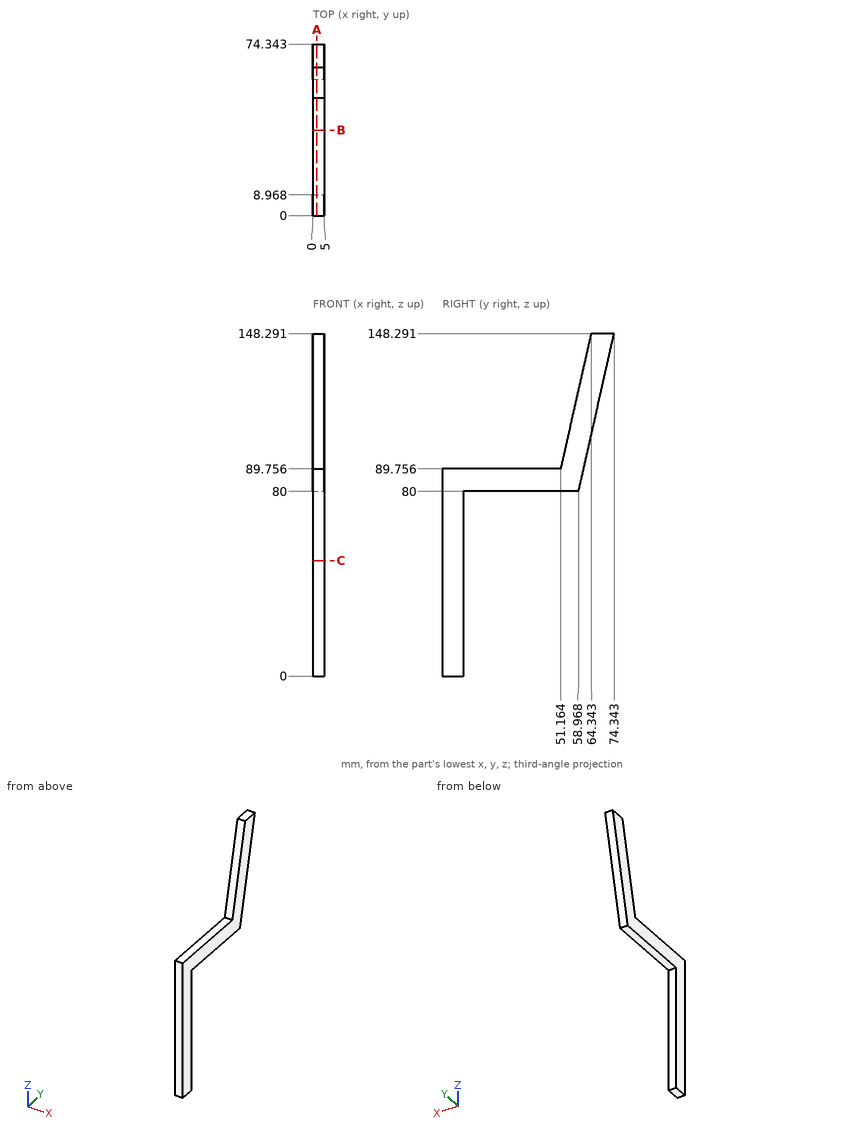
Study the drawing (mm; zero at the part's minimum x, y, z) and answer. Coordinates: 2 decimals unless noted, no trailing zeros. Loops run counter-clockwise (first coordinate to the right, second up) from the corner with the lowest first, then second, coordinate; pieces in that order, holes last. Notation, with made-up numbers: M 5.25,-6 L 37.25,-6 A22 cw 37.25,20 Z; hole C -23,-13.5 d2. An arc over 180 degrees is marked long. Answer in a Markdown table with one row per item.
1) Given pin 1 (1.5 mm diameter, centred on x = 1, z = 126, fed in from +Y), flat-ended and moving along its own axis, determine where the tip first touches the part or whether it passes through.
Answers below:
| item | result |
|---|---|
| pin 1 | y = 69.49 |
2) Find the intervals of material crossed by probe 1 along Z at (x, y) = (4.55, 48) (1 decimal); probe 2 along Y at (x, z) = (0.55, 59); probe 3 along Y at (x, z) = (0.3, 108), in increasing order.
Answers below:
| item | result |
|---|---|
| probe 1 | 80 to 89.8 |
| probe 2 | 0 to 8.97 |
| probe 3 | 55.27 to 65.27 |
3) Find section A-A (x = 1.7). Determine the outline of the cut face in (y, z) (1 decimal).
Answers below:
| item | result |
|---|---|
| outline | M 0,0 L 9,0 L 9,80 L 59,80 L 74.3,148.3 L 64.3,148.3 L 51.2,89.8 L 0,89.8 Z |
4) Find section B-B (y = 37). Determine the outline of the cut face in (x, z) (1 decimal), then the cut area to 3 significant figures.
Answers below:
| item | result |
|---|---|
| outline | M 0,80 L 5,80 L 5,89.8 L 0,89.8 Z |
| area | 48.8 mm^2 |
5) Find section C-C (z = 50). Determine the outline of the cut face in (x, y).
Answers below:
| item | result |
|---|---|
| outline | M 0,0 L 5,0 L 5,8.97 L 0,8.97 Z |
